```python
from build123d import *

# Parameters (mm, degrees)
BOSS_EXTRUDE2_DEPTH = 15
BOSS_EXTRUDE3_START = -3
BOSS_EXTRUDE3_DEPTH = 3


with BuildPart() as part:
    # Sketch1 → Boss-Extrude2 (new body)
    with BuildSketch(Plane(origin=(0, 0, 0), x_dir=(1, 0, 0), z_dir=(0, 1, 0))):
        with BuildLine():
            ThreePointArc((-85.5, -45.5), (-89.035533906, -44.035533906), (-90.5, -40.5))
            Line((-90.5, -40.5), (-90.5, 35.668613654))
            ThreePointArc((-90.5, 35.668613654), (-89.065520601, 39.113080167), (-87.5, 42.5))
            Line((-87.5, 42.5), (-87.5, -42.5))
            Line((-87.5, -42.5), (87.5, -42.5))
            Line((87.5, -42.5), (87.5, 42.5))
            ThreePointArc((87.5, 42.5), (89.065520601, 39.113080167), (90.5, 35.668613654))
            Line((90.5, 35.668613654), (90.5, -40.5))
            ThreePointArc((90.5, -40.5), (89.035533906, -44.035533906), (85.5, -45.5))
            Line((85.5, -45.5), (-85.5, -45.5))
        make_face()
    extrude(amount=BOSS_EXTRUDE2_DEPTH)

    # Sketch3 → Boss-Extrude3 (add)
    with BuildSketch(Plane(origin=(0, 0, 0), x_dir=(1, 0, 0), z_dir=(0, 1, 0)).offset(BOSS_EXTRUDE3_START)):
        with BuildLine():
            Line((87.5, 42.5), (-12.5, 42.5))
            Line((-12.5, 42.5), (-12.5, -45.5))
            Line((-12.5, -45.5), (85.5, -45.5))
            ThreePointArc((85.5, -45.5), (89.035533906, -44.035533906), (90.5, -40.5))
            Line((90.5, -40.5), (90.5, 35.668613654))
            Line((90.5, 35.668613654), (87.5, 42.5))
        make_face()
    extrude(amount=BOSS_EXTRUDE3_DEPTH)


solid = part.part
```
Could you check a few things on this model? Use its own coordinates, in mm. A direction names the side the tool comes from. Round coordinates to 2 decimals unless told otherwise and drop trailing zeros. Order: outer loops, then holes, each group sorted by start corner. A loop starts at its lowest first (then second) coordinate and runs counter-clockwise, first axis right, second up. Notation, with made-up numbers: M 68.25,12.5 L 121.25,12.5 A13 cw 121.25,19.5 Z; hole C 73,22 d4. An arc over 180 degrees is marked long. One line per question, with ' | ' between items. Start each with the question number.
(1) Suppose I cut it at A-A on z = -2. List the corners of the cut face in (x, y) for me, then the cut area to 3 significant figures.
(2) For P1, Ø1.5, axis at x = -9.5, y = 11.5, coming from the -Z side; P2, Ø5, axis at x = 28.5, z = -19.5, coming from the +Y side; P3, Ø0.9, axis at y = -1.5, z = -12, coming from the -X side, each with a flat end and sliding along its axis, tell me the tip position at first contact or that it passes through.
(3) For faces 1 (the face through (37, 0, -1)), 2 (the face through (-87.5, 7, -1)), 3 (the face through (89.045, 7.395, -39.161)), which set-ups out of +Z, -Z, +X, -X, +Y, -Y let a thin tool reach every point of the face, with its end or its side?
(4) Suppose I cut it at D-D on x = -29. List the corners of the cut face in (y, z) for me.
(5) Suppose I cut it at C-C on x = 50. List the corners of the cut face in (y, z) for me.
(6) Thinking about a two-plate mould opening in X: for faces 4 (the face through (-89, 0, 24)), 5 (the face through (-1, 7, 42.5)), 6 (the face through (-90.5, 7, 3)), 7 (the face through (87.5, 7, 1)), which applies, +X half, -X half, draft (parallel to the pull), parting line (faces both ways), or undercut?
(7) Suppose I cut it at B-B on y = 2. List the corners of the cut face in (x, z) for me, then the cut area to 3 significant figures.
(8) Please list where these lines run through material, in increasing order: line 1 along X through (y, z) = (8.75, 9.5); line 2 along X through (y, z) = (-0.75, -10.5); line 3 along Y through (x, z) = (-2, -35).
Geometry results:
1) outline: M -90.5,0 L -87.5,0 L -87.5,15 L -90.5,15 Z; M -12.5,-3 L 90.5,-3 L 90.5,15 L 87.5,15 L 87.5,0 L -12.5,0 Z | area: 399 mm²
2) P1: z = 42.5 | P2: y = 0 | P3: x = -12.5
3) face 1: -Z, +Y | face 2: -Z, +Y, -Y | face 3: -Z, +X, +Y, -Y
4) outline: M 0,42.5 L 15,42.5 L 15,45.5 L 0,45.5 Z
5) outline: M -3,-42.5 L 0,-42.5 L 0,42.5 L 15,42.5 L 15,45.5 L -3,45.5 Z
6) face 4: draft | face 5: undercut | face 6: -X half | face 7: undercut
7) outline: M -90.5,-35.67 A97.28 ccw -87.5,-42.5 L -87.5,42.5 L 87.5,42.5 L 87.5,-42.5 A97.28 ccw 90.5,-35.67 L 90.5,40.5 A5 ccw 85.5,45.5 L -85.5,45.5 A5 ccw -90.5,40.5 Z | area: 1,020 mm²
8) line 1: -90.5 to -87.5, 87.5 to 90.5 | line 2: -12.5 to 90.5 | line 3: -3 to 0
